The model under review builds one solid part; all positions refer to its coordinate system, in mm. A direction names the side the tool comes from. Give positions to 0.01 mm unless a question says otherwise; leave off trailing zeros. Loops run counter-clockwise (first coordinate to the right, second up) from the corner with the lowest first, then second, coordinate; pieces in that order, holes last. Notation, with made-up numbers: M 1.5,36.25 L 8.5,36.25 A21 cw 8.5,60.25 Z; hole C 21,13 d7. An arc over 180 degrees is marked long. Return JSON: item names as keys, results as strings.
```python
from build123d import *

# Parameters (mm, degrees)
SKETCH1_R           = 1.25
BOSS_EXTRUDE1_DEPTH = 13.8
SKETCH3_R           = 2
BOSS_EXTRUDE2_DEPTH = 0.01
DOME1_FACE_RADIUS   = 2
DOME1_HEIGHT        = 1
SCALE1_SCALE        = 1.5


with BuildPart() as part:
    # Sketch1 → Boss-Extrude1 (new body)
    with BuildSketch(Plane.XY):
        Circle(SKETCH1_R)
    extrude(amount=BOSS_EXTRUDE1_DEPTH)

    # Sketch3 → Boss-Extrude2 (add)
    with BuildSketch(Plane(origin=(0, 0, 0), x_dir=(-1, 0, 0), z_dir=(0, 0, -1))):
        with Locations(Location((0, 0, 0), (0, 0, 180))):
            Circle(SKETCH3_R)
    extrude(amount=BOSS_EXTRUDE2_DEPTH)

    # Dome1: a dome of height H over a round flat face of radius A is a cap of a sphere of radius (A * A + H * H) / (2 * H)
    dome1_r = (DOME1_FACE_RADIUS * DOME1_FACE_RADIUS + DOME1_HEIGHT * DOME1_HEIGHT) / (2 * DOME1_HEIGHT)
    dome1_base = Plane((0, 0, -0.01), z_dir=(0, 0, -1))
    with Locations(dome1_base.offset(DOME1_HEIGHT - dome1_r)):
        dome1_ball = Sphere(dome1_r, mode=Mode.PRIVATE)
    add(split(dome1_ball, bisect_by=dome1_base, keep=Keep.TOP, mode=Mode.PRIVATE))


with BuildPart() as part_1:
    # Scale1: scaled about (0, 0, 6.226948778)
    add(part.part.scale(SCALE1_SCALE).moved(Location((0, 0, -3.113474389))))


solid = part_1.part
```
1) Tool access review of faces 1 (the face through (-1.873, 0.082, 7.092)), 2 (the face through (0, 0, 17.587)): name each direction out of +Z, -Z, +X, -X, +Y, -Y from which nothing blocks a thin tool from reaching the whole face with its end or side.
From the geometry:
{"face 1": "+Z", "face 2": "+Z, +X, -X, +Y, -Y"}
2) Wall thickness on L1, parallel to X at y = -0.05, z = 13.5; L2, parallel to Z at x = 1.5, y = -2.4; L3, parallel to X at y = -1.25, z = 14.5: over which ranges is each line inside the solid? List them lowest first. Write a range as from..to.
From the geometry:
{"L1": "-1.87..1.87", "L2": "-3.34..-3.11", "L3": "-1.4..1.4"}
3) Consider section C-C on z = 16.25. Write out the cut boundary in (x, y) (3 decimals).
From the geometry:
{"outline": "C 0,0 d3.75"}
4) Consider section A-A on x = 0. Write out the cut boundary in (y, z) (3 decimals).
From the geometry:
{"outline": "M -3,-3.128 A3.75 ccw 3,-3.128 L 3,-3.113 L 1.875,-3.113 L 1.875,17.587 L -1.875,17.587 L -1.875,-3.113 L -3,-3.113 Z"}
5) Insertion check: pin 1 (2 mm diameter, centred on x = 2.5, z = 14.5, fed in from +Y) (3 decimals); pin 2 (1 mm diameter, centred on x = -0.5, y = -2, fed in from -Z); pin 3 (3 mm diameter, centred on x = -1, z = 2.5, fed in from -Y) (3 decimals). Each pin has a flat end and moves straight along its axis. Give the tip position at first contact, or say it passes through.
From the geometry:
{"pin 1": "y = 1.125", "pin 2": "z = -4.29", "pin 3": "y = -1.875"}
